Input: part model. Units: mm. Frame: model coordinates. Face numbers are marked on the shaded views. Coordinates: 2 decimals unless noted, no trailing zeros. Write each loop counter-clockwise with the first axis right and the second up, starting at its lowest first coordinate (ties: lowest second). Pieces come first, ordered by that corner, then holes. Notation, with made-up numbers: (69, -34.75) - (92, -34.75) arc R23 ccw to (92, -14.75) - close; hole circle Ø11 at (-20.5, 28.25). An arc over 180 degrees is marked (long way). Use a Markdown table: item, result. Add a question column.
Q1. Material intervals for probe 1 along Y at (x, z) = (-65.9, 0); probe 2 along Y at (x, z) = (-25.5, 0) (3 decimals); probe 3 along Z at (x, y) = (-51, -0.5), sorted ascending. Write a range as from..to.
Q2. Section query A-A (z = 0). Return the cut outline in (x, y) (1 decimal), then the cut area to 3 significant figures.
Q3. Section query C-C (x = -32). Return the cut outline in (y, z) (3 decimals), then the cut area to 3 significant figures.
Q4. Pin query (flat end, axial travel): P1, Ø3, axis at x = -40, y = -7, coming from the +Z side; P2, Ø2, axis at x = -15.5, y = 4.5, coming from the -Z side; P3, Ø5, axis at y = 3, z = 0, coming from the -X side. Return the tip coordinate at first contact, or that it passes through.
Q5. Mould query, pull axis Z, two halves, no side actions, for the marked faces 1, 2 and 3. Classes: released by +Z, released by -Z, zero draft, split by the parting line, or undercut.
from build123d import *


with BuildPart() as part:
    # Sketch1 → Revolve1 (revolve)
    with BuildSketch(Plane(origin=(0, 0, 0), x_dir=(1, 0, 0), z_dir=(0, 1, 0))):
        with BuildLine():
            Line((0, 0), (3.175, 0))
            Line((3.175, 0), (3.175, 11.176))
            ThreePointArc((3.175, 11.176), (2.728630735, 12.253630735), (1.651, 12.7))
            Line((1.651, 12.7), (-66.675, 12.7))
            Line((-66.675, 12.7), (-66.675, 11.1125))
            Line((-66.675, 11.1125), (-65.0748, 11.1125))
            Line((-65.0748, 11.1125), (-65.0748, 9.525))
            Line((-65.0748, 9.525), (-1.524, 9.525))
            ThreePointArc((-1.524, 9.525), (-0.446369265, 9.078630735), (0, 8.001))
            Line((0, 8.001), (0, 0))
        make_face()
    revolve(axis=Axis((0, 0, 0), (1, 0, 0)))


solid = part.part
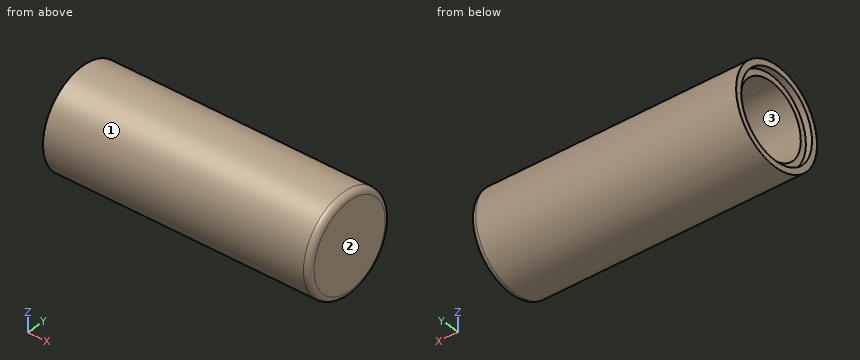
Values follow:
| question | item | result |
|---|---|---|
| 1 | probe 1 | -12.7..-11.11, 11.11..12.7 |
| 1 | probe 2 | -12.7..-9.525, 9.525..12.7 |
| 1 | probe 3 | -12.69..-9.51, 9.51..12.69 |
| 2 | outline | (-66.7, -12.7) - (1.7, -12.7) arc R1.5 ccw to (3.2, -11.2) - (3.2, 11.2) arc R1.5 ccw to (1.7, 12.7) - (-66.7, 12.7) - (-66.7, 11.1) - (-65.1, 11.1) - (-65.1, 9.5) - (-1.5, 9.5) arc R1.5 cw to (0, 8) - (0, -8) arc R1.5 cw to (-1.5, -9.5) - (-65.1, -9.5) - (-65.1, -11.1) - (-66.7, -11.1) - close |
| 2 | area | 499 mm2 |
| 3 | outline | circle Ø25.4 at (0, 0); hole circle Ø19.05 at (0, 0) |
| 3 | area | 222 mm2 |
| 4 | P1 | z = 11.45 |
| 4 | P2 | z = -12.21 |
| 4 | P3 | x = 0 |
| 5 | face 1 | split by the parting line |
| 5 | face 2 | zero draft |
| 5 | face 3 | undercut |
